Could you check a few things on this model? Use its own coordinates, in mm. A direction names the side the tool comes from. Give positions to 0.01 mm unless a question says otherwise; leave off trailing zeros. Order: outer loops, then holes, each group sorted by start corner. A loop starts at its lowest first (then second) coordinate and runs counter-clockwise, first axis right, second up. Notation, with made-up numbers: M 23.5,87 L 47.5,87 A21 ccw 47.5,113 Z; hole C 28.5,-30.75 d1. An arc over 180 degrees is marked long. Use a Markdown table: item, result. Add a question column.
Item 1: Suppose I cut it at B-B on x = 75. Write out the boundary of the cut face in (y, z), plus the area to 3 significant figures.
Item 2: For faces 1 (the face through (-11, -32, 2)), 2 (the face through (-59.5, -8, 9)), 3 (the face through (-11, -27.5, 12)), 4 (the face through (-11, 12.5, 12)), which set-ups out of +Z, -Z, +X, -X, +Y, -Y let a thin tool reach every point of the face, with its end or its side?
Item 3: Suppose I cut it at A-A on y = -25. Write out the boundary of the cut face in (x, z), plus the area to 3 significant figures.
Item 4: I'm going to push flat-ended pins straight in: pin 1 Ø2.5 at (x, y) = (11, 15.5) entering from +Z; pin 2 Ø2.5 at (x, z) = (-3.5, 4) entering from +Y; pin 3 Ø4 at (x, y) = (-75, -25) entering from +Z. Where does each tip first touch, or does it pass through?
Item 5: Suppose I cut it at C-C on x = 6. Write out the boundary of the cut face in (y, z), plus the area to 3 significant figures.
Item 6: If we mould it in two halves opening along X, with no side actions, what happens to faces 5 (the face through (-11, 21.012, 4)), 6 (the face through (76.669, -24.474, 0.986)), 7 (the face through (38.5, -9, 9))? For each: released by +X, released by -X, zero draft, split by the parting line, or undercut.
Item 7: Suppose I cut it at D-D on z = 5.5. Write out the boundary of the cut face in (x, y).
Item 8: If I drill on L1, parallel to Y at x = 75, z = 1.25; L2, parallel to Y at x = 30, z = 3; L3, parallel to Y at x = -8.5, z = 1, over which ranges is the centre line in solid material (lowest first)? Write a range as from..to.
from build123d import *

# Parameters (mm, degrees)
F0_W     = 155
F0_H     = 55
F0_R     = 1.75
F1_DEPTH = 2
F2_W     = 98
F2_H     = 48.51198
F2_H_2   = 10
F3_DEPTH = 5
F4_W     = 98
F4_H     = 40
F5_DEPTH = 10


with BuildPart() as f1:
    # F0 (on Top) → F1 (new body)
    with BuildSketch(Plane.XY):
        Rectangle(F0_W, F0_H)
        with Locations((-75, -25)):
            Circle(F0_R, mode=Mode.SUBTRACT)
        with Locations((75, -25)):
            Circle(F0_R, mode=Mode.SUBTRACT)
        with Locations((-75, 25)):
            Circle(F0_R, mode=Mode.SUBTRACT)
        with Locations((75, 25)):
            Circle(F0_R, mode=Mode.SUBTRACT)
    extrude(amount=F1_DEPTH)

    # F2 (on face) → F3 (join)
    with BuildSketch(Plane.XY.offset(2)):
        with Locations((-10.5, -3.24401)):
            Rectangle(F2_W, F2_H)
        with Locations((-10.5, -32.5)):
            Rectangle(F2_W, F2_H_2)
    extrude(amount=F3_DEPTH)

    # F4 (on face) → F5 (join)
    with BuildSketch(Plane.XY.offset(7)):
        with Locations((-10.5, -7.5)):
            Rectangle(F4_W, F4_H)
    extrude(amount=F5_DEPTH)


solid = f1.part
Findings below:
| question | item | result |
|---|---|---|
| 1 | outline | M -27.5,0 L -26.75,0 L -26.75,2 L -27.5,2 Z; M -23.25,0 L 23.25,0 L 23.25,2 L -23.25,2 Z; M 26.75,0 L 27.5,0 L 27.5,2 L 26.75,2 Z |
| 1 | area | 96.0 mm^2 |
| 2 | face 1 | -Z, +X, -X, -Y |
| 2 | face 2 | +Z, -X, +Y, -Y |
| 2 | face 3 | +Z, +X, -X, -Y |
| 2 | face 4 | +Z, +X, -X, +Y |
| 3 | outline | M -77.5,0 L -76.75,0 L -76.75,2 L -77.5,2 Z; M -73.25,0 L 73.25,0 L 73.25,2 L 38.5,2 L 38.5,17 L -59.5,17 L -59.5,2 L -73.25,2 Z; M 76.75,0 L 77.5,0 L 77.5,2 L 76.75,2 Z |
| 3 | area | 1,770 mm^2 |
| 4 | pin 1 | stops at z = 7 |
| 4 | pin 2 | stops at y = 21.01 |
| 4 | pin 3 | stops at z = 2 |
| 5 | outline | M -37.5,2 L -27.5,2 L -27.5,0 L 27.5,0 L 27.5,2 L 21.01,2 L 21.01,7 L 12.5,7 L 12.5,17 L -27.5,17 L -27.5,7 L -37.5,7 Z |
| 5 | area | 803 mm^2 |
| 6 | face 5 | zero draft |
| 6 | face 6 | undercut |
| 6 | face 7 | released by +X |
| 7 | outline | M -59.5,-37.5 L 38.5,-37.5 L 38.5,21.01 L -59.5,21.01 Z |
| 8 | L1 | y = -27.5..-26.75, -23.25..23.25, 26.75..27.5 |
| 8 | L2 | y = -37.5..21.01 |
| 8 | L3 | y = -27.5..27.5 |
